Check sheet for the modelled part. Datum: model origin and axes. Units: mm. A direction names the side the tool comes from. Round coordinates to 2 decimals unless told otherwise and drop trailing zeros. Loops run counter-clockwise (first coordinate to the right, second up) from the corner with the lowest first, then second, coordinate; pieces in that order, holes last. Notation, with made-up numbers: (13, 88) -> (30, 88) arc R21 ccw to (30, 120) -> close; hole circle Ø11 at (2.5, -16.5). An arc over 180 degrees is marked (long way). Return JSON: item names as keys, results as strings.
from build123d import *

# Parameters (mm, degrees)
F0_R      = 6
F1_DEPTH  = 30
F6_R      = 4.25
F8_DEPTH  = 13.262673
F7_R      = 4.25
F9_DEPTH  = 13.262673
F3_R      = 4.25
F10_DEPTH = 12.001


with BuildPart() as f1:
    # F0 (on Front) → F1 (new body)
    with BuildSketch(Plane.XZ):
        Circle(F0_R)
    extrude(amount=F1_DEPTH)

    # F6 (on face) → F8 (cut, through all)
    with BuildSketch(Plane(origin=(0, 0.407003, -4.652062), x_dir=(1, 0, 0), z_dir=(0, 0.087156, -0.996195))):
        with Locations((0, 15.465855)):
            Circle(F6_R)
    extrude(amount=-F8_DEPTH, mode=Mode.SUBTRACT)

    # F7 (on face) → F9 (cut, through all)
    with BuildSketch(Plane(origin=(0, -0.634886, -7.256785), x_dir=(1, 0, 0), z_dir=(0, -0.087156, -0.996195))):
        with Locations((0, 14.419986)):
            Circle(F7_R)
    extrude(amount=-F9_DEPTH, mode=Mode.SUBTRACT)

    # F3 (on offset) → F10 (cut, through all)
    with BuildSketch(Plane.XY.offset(-6)):
        with Locations((0, -15)):
            Circle(F3_R)
    extrude(amount=F10_DEPTH, mode=Mode.SUBTRACT)


solid = f1.part
Q1. Section check C-C (y = -21.5). Record the boundary of the cut face in (x, z), then the cut area to 3 significant figures.
Results list:
{"outline": "circle Ø12 at (0, 0)", "area": "113 mm^2"}
Q2. Draft check along X on faces 3 (the cylindrical face through (0.1, -19.783, -0.084)), 4 (the cylindrical face through (4.25, -15.01, 0.9)), 5 (the cylindrical face through (-4.76, -14.79, -3.65)), 6 (the flat face through (0, -30, 0)). Enter one of: released by +X, released by -X, zero draft, split by the parting line, or undercut.
Results list:
{"face 3": "undercut", "face 4": "undercut", "face 5": "split by the parting line", "face 6": "zero draft"}
Q3. Tool access check on faces 1 (the cylindrical face through (-4.25, -14.99, 0.9)), 2 (the flat face through (0, 0, 0)). Record the directions out of +Z, -Z, +X, -X, +Y, -Y that give a thin tool (end or side, any length) a straight path to the whole face; none if there is none.
Results list:
{"face 1": "+Z, -Z", "face 2": "+Z, -Z, +X, -X, +Y"}
Q4. Section check A-A (x = -1.75). Record the boundary of the cut face in (y, z), then the cut area to 3 significant figures.
Results list:
{"outline": "(-30, -5.74) -> (-18.91, -5.74) -> (-19.91, 5.74) -> (-30, 5.74) -> close; (-11.09, -5.74) -> (0, -5.74) -> (0, 5.74) -> (-10.09, 5.74) -> close", "area": "243 mm^2"}
Q5. Material ranges on line 1 (Y direction, x = -3.5, z = 4); line 2 (Y direction, x = 0.5, z = -4); line 3 (X direction, y = -14.5, z = -0.25), recorded low to high.
Results list:
{"line 1": "-30 to -18.3, -11.7 to 0", "line 2": "-30 to -19.41, -10.59 to 0", "line 3": "-5.99 to -4.25, 4.25 to 5.99"}
Q6. Go/stop test with flat-tipped pins: pin 1 (6 mm diameter, centred on x = 2, y = -13, fed in from +Z); pin 2 (1 mm diameter, centred on y = -11.5, z = 1, fed in from -X). Record where each tip stops, or that it passes through.
Results list:
{"pin 1": "z = 5.78", "pin 2": "x = -5.98"}
Q7. Section check B-B (x = 0). Record the boundary of the cut face in (y, z), then the cut area to 3 significant figures.
Results list:
{"outline": "(-30, -6) -> (-19.27, -6) -> (-20.32, 6) -> (-30, 6) -> close; (-10.73, -6) -> (0, -6) -> (0, 6) -> (-9.68, 6) -> close", "area": "245 mm^2"}
